from build123d import *

# Parameters (mm, degrees)
SKETCH2_W           = 15
SKETCH2_H           = 93.194890567
BOSS_EXTRUDE2_DEPTH = 50
SKETCH3_R           = 9
CUT_EXTRUDE6_DEPTH  = 105
BOSS_EXTRUDE4_DEPTH = 50
SKETCH7_R           = 6.5
CUT_EXTRUDE7_DEPTH  = 105
SKETCH8_R           = 20
CUT_EXTRUDE8_DEPTH  = 235
SKETCH11_W          = 15
SKETCH11_H          = 40
BOSS_EXTRUDE5_DEPTH = 60
SKETCH12_R          = 11
CUT_EXTRUDE9_DEPTH  = 60


with BuildPart() as part:
    # Sketch1 → Revolve1 (revolve)
    with BuildSketch(Plane.XY):
        Polygon((0, 260), (30, 260), (30, 250), (22.65711135, 250), (35, 180), (35, 130), (25, 130), (25, 50), (35, 50), (35, 0), (0, 0), align=None)
    revolve(axis=Axis((0, 462.148353897, 0), (0, -1, 0)))

    # Sketch2 → Boss-Extrude2 (add)
    with BuildSketch(Plane(origin=(0, 0, 0), x_dir=(1, 0, 0), z_dir=(0, 1, 0))):
        with Locations((-27.5, -46.597445284)):
            Rectangle(SKETCH2_W, SKETCH2_H)
        with Locations((27.5, -46.597445284)):
            Rectangle(SKETCH2_W, SKETCH2_H)
    extrude(amount=BOSS_EXTRUDE2_DEPTH)

    # Sketch3 → Cut-Extrude6 (cut)
    with BuildSketch(Plane.ZY.offset(35)):
        with Locations((48, 19)):
            Circle(SKETCH3_R)
        with BuildLine():
            Line((73.603646545, 27.287280664), (41.166521698, 50))
            Line((41.166521698, 50), (93.194890567, 50))
            Line((93.194890567, 50), (93.194890567, 0))
            Line((93.194890567, 0), (65, 0))
            ThreePointArc((65, 0), (79.305754261, 10.489413007), (73.603646545, 27.287280664))
        make_face()
    extrude(amount=-CUT_EXTRUDE6_DEPTH, mode=Mode.SUBTRACT)

    # Sketch6 → Boss-Extrude4 (add)
    with BuildSketch(Plane(origin=(0, 180, 0), x_dir=(1, 0, 0), z_dir=(0, 1, 0))):
        Polygon((0, 0), (7.5, 0), (7.5, -91.66287292), (-7.5, -91.66287292), (-7.5, 0), align=None)
        Polygon((7.5, 91.66287292), (7.5, 9.253142795), (-7.5, 9.974305291), (-7.5, 91.66287292), align=None)
    extrude(amount=-BOSS_EXTRUDE4_DEPTH)

    # Sketch7 → Cut-Extrude7 (cut)
    with BuildSketch(Plane.ZY.offset(7.5)):
        with BuildLine():
            ThreePointArc((-83.531871553, 152.480329712), (-89.300855909, 138.980393779), (-77.686985828, 130))
            Line((-77.686985828, 130), (-91.66287292, 130))
            Line((-91.66287292, 130), (-91.66287292, 180))
            Line((-91.66287292, 180), (-37.731448931, 180))
            Line((-37.731448931, 180), (-83.531871553, 152.480329712))
        make_face()
        with BuildLine():
            Line((34.186985828, 180), (34.186985828, 178.231443671))
            Line((34.186985828, 178.231443671), (77.367442727, 152.286007608))
            ThreePointArc((77.367442727, 152.286007608), (82.750551266, 138.793139487), (71.186985828, 130))
            Line((71.186985828, 130), (91.66287292, 130))
            Line((91.66287292, 130), (91.66287292, 180))
            Line((91.66287292, 180), (34.186985828, 180))
        make_face()
        with Locations((54.186985828, 144.29)):
            Circle(SKETCH7_R)
        with Locations((-59.186985828, 142)):
            Circle(SKETCH7_R)
    extrude(amount=-CUT_EXTRUDE7_DEPTH, mode=Mode.SUBTRACT)

    # Sketch8 → Cut-Extrude8 (cut)
    with BuildSketch(Plane.XZ):
        Circle(SKETCH8_R)
    extrude(amount=-CUT_EXTRUDE8_DEPTH, mode=Mode.SUBTRACT)

    # Sketch11 → Boss-Extrude5 (add)
    with BuildSketch(Plane(origin=(0, 260, 0), x_dir=(1, 0, 0), z_dir=(0, 1, 0))):
        with Locations((-10, 0)):
            Rectangle(SKETCH11_W, SKETCH11_H)
    extrude(amount=BOSS_EXTRUDE5_DEPTH)

    # Sketch12 → Cut-Extrude9 (cut)
    with BuildSketch(Plane.ZY.offset(17.5)):
        with Locations((0, 290)):
            Circle(SKETCH12_R)
        with BuildLine():
            Line((-20, 290), (-20, 320))
            Line((-20, 320), (20, 320))
            Line((20, 320), (20, 290))
            ThreePointArc((20, 290), (0, 310), (-20, 290))
        make_face()
    extrude(amount=-CUT_EXTRUDE9_DEPTH, mode=Mode.SUBTRACT)


solid = part.part
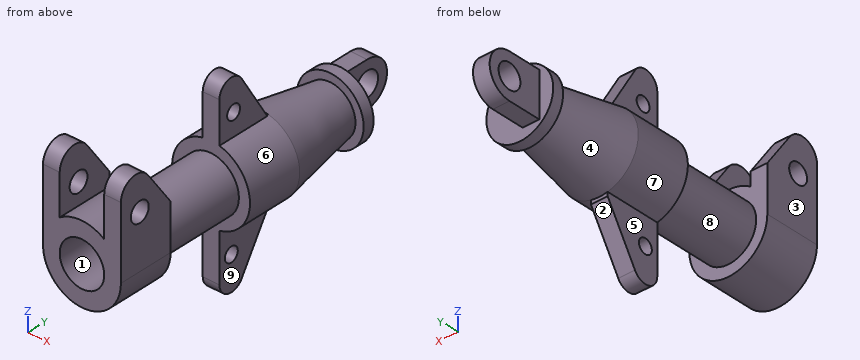
Geometry: final body of the model. Coordinates: model frame, mm. Face numbers are marked on the shaded views. A direction names the side the tool comes from. Give positions to 0.01 mm unless a question says otherwise; leave off trailing zeros. Write each loop counter-clockwise with the first axis right and the second up, starting at its lowest first coordinate (ties: lowest second). Pieces come first, ordered by that corner, then holes. Notation, with made-up numbers: (-10, -16.75) - (34, -16.75) arc R13 ccw to (34, -8.75) - close; hole circle Ø5 at (29, 89.5). An arc over 180 degrees is marked (long way). Return JSON: item names as keys, results as strings. Group by question number.
1) Section A-A on y = 19. Return the cut outline in (x, z), plus the area to 3 significant figures.
2) Mould query, pull axis X, two halves, no side actions, for the marked faces 1, 2, 3 and 4. Classes: released by +X, released by -X, zero draft, split by the parting line, or undercut.
3) Line query: line 1 (Z direction, x = 0.5, y = 56) (3 decimals); line 2 (Y direction, x = 32.5, z = 34); line 3 (Z direction, x = -9.5, y = 268). Output: solid intervals per line, ascending.
4) Set-up query: the marked faces 5, 6, 7, 8 and 9. Return all of +Z, -Z, +X, -X, +Y, -Y with unobstructed straight access to the full face (end or side cutting, diameter ignored); none if empty.
5) First-contact query: P1, Ø12, axis at y = 155.5, z = 44, coming from the +X side; P2, Ø3, axis at x = -24, y = 149, coming from the -Z side; P3, Ø5, axis at x = -2, z = 18.5, coming from the +Y side. Flat tips, straight axial feed; report the tip coordinate or a pass-through.
6) Section C-C on y = 231.5. Return the cut outline in (x, z), plus the area to 3 significant figures.
7) Section B-B on z = -59. Return the cut outline in (x, y).
Filled in:
{
 "1": {"outline": "(-35, 0) arc R35 ccw to (35, 0) - (35, 39) - (20, 39) - (20, 28.72) arc R35 ccw to (-20, 28.72) - (-20, 39) - (-35, 39) - close; (-35, 57) - (-20, 57) - (-20, 79.46) - (-35, 79.46) - close; (20, 57) - (35, 57) - (35, 79.46) - (20, 79.46) - close; hole circle Ø40 at (0, 0)", "area": "3,830 mm^2"},
 "2": {"face 1": "undercut", "face 2": "zero draft", "face 3": "released by -X", "face 4": "split by the parting line"},
 "3": {"line 1": "z = -24.995 to -19.994, 19.994 to 24.995", "line 2": "y = 0 to 50", "line 3": "z = -20 to 20"},
 "4": {"face 5": "-Z, -X, +Y, -Y", "face 6": "+X, +Y", "face 7": "-X, +Y", "face 8": "none", "face 9": "-Z, +X, +Y, -Y"},
 "5": {"P1": "stops at x = 7.5", "P2": "stops at z = -26.81", "P3": "stops at y = 301.93"},
 "6": {"outline": "circle Ø51.84 at (0, 0); hole circle Ø40 at (0, 0)", "area": "854 mm^2"},
 "7": {"outline": "(-7.5, 130) - (7.5, 130) - (7.5, 135.5) - (-7.5, 135.5) - close; (-7.5, 148.5) - (7.5, 148.5) - (7.5, 167.22) - (-7.5, 167.22) - close"}
}
